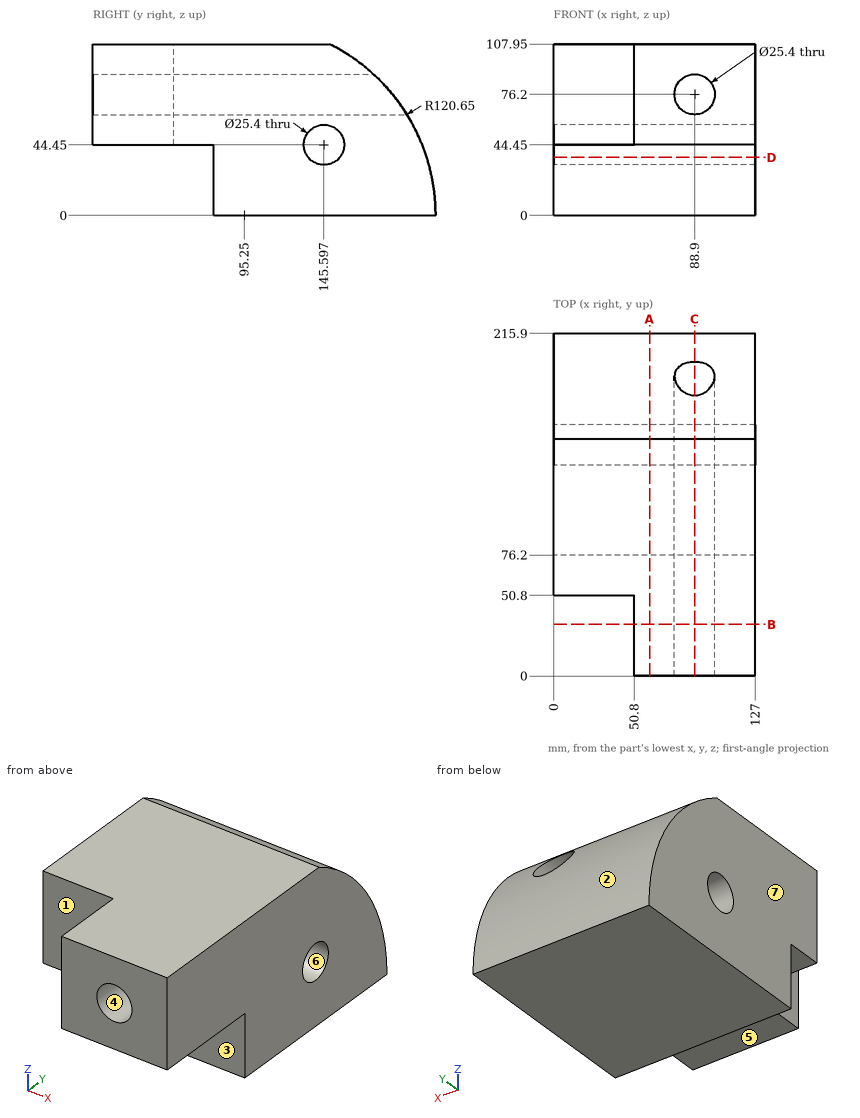
Job drawing, mm, ordinate dimensions from the low corner. One solid piece. A direction names the side the tool comes from. Round coordinates to 2 decimals unless told otherwise and drop trailing zeros. Order: outer loops, then holes, each group sorted by start corner. A loop starts at its lowest first (then second) coordinate and runs counter-clockwise, first axis right, second up. Notation, with made-up numbers: (-22, 54.25) -> (12, 54.25) arc R21 cw to (12, 61.25) -> close; hole circle Ø7 at (-5.5, -36). An arc over 180 degrees is marked (long way). Answer in a Markdown table with one row per item.
1) Mould opens along Z. For the marked faces 4, 5, 6 and 7 say: released by +Z, released by -Z, zero draft, split by the parting line, or undercut.
Values:
| item | result |
|---|---|
| face 4 | undercut |
| face 5 | released by -Z |
| face 6 | undercut |
| face 7 | zero draft |
2) Band-saw the part on A-A on x = 60.5. Give the cut face in (y, z).
Values:
| item | result |
|---|---|
| outline | (0, 44.45) -> (76.2, 44.45) -> (76.2, 0) -> (215.9, 0) arc R120.65 ccw to (149.13, 107.95) -> (0, 107.95) -> close; hole circle Ø25.4 at (145.6, 44.45) |
3) Band-saw the part on C-C on x = 88.9. Give the cut face in (y, z).
Values:
| item | result |
|---|---|
| outline | (0, 44.45) -> (76.2, 44.45) -> (76.2, 0) -> (215.9, 0) arc R120.65 ccw to (197.84, 63.5) -> (0, 63.5) -> close; (0, 88.9) -> (176.82, 88.9) arc R120.65 ccw to (149.13, 107.95) -> (0, 107.95) -> close; hole circle Ø25.4 at (145.6, 44.45) |
4) Band-saw the part on D-D on z = 36.5. Give the cut face in (x, y), and give its area (3 significant figures).
Values:
| item | result |
|---|---|
| outline | (0, 76.2) -> (127, 76.2) -> (127, 135.69) -> (0, 135.69) -> close; (0, 155.5) -> (127, 155.5) -> (127, 210.25) -> (0, 210.25) -> close |
| area | 14,500 mm2 |
5) Which spindle directions (+Z, -Z, +X, -X, +Y, -Y) get a long thin tool onto all of the face, cutting with end or side? Do the marked faces 1, 2 and 3. Say none if no direction does.
Values:
| item | result |
|---|---|
| face 1 | +Z, -Z, -X, -Y |
| face 2 | +Z, +X, -X, +Y |
| face 3 | -Z, +X, -X, -Y |
6) Wall check: L1, parallel to Z at x = 88.9, y = 114.5; L2, parallel to X at y = 25, z = 54.5; L3, parallel to X at y = 14, z = 69. Give the ranges that are in metal, low to high.
Values:
| item | result |
|---|---|
| L1 | 0 to 63.5, 88.9 to 107.95 |
| L2 | 50.8 to 127 |
| L3 | 50.8 to 78.44, 99.36 to 127 |
7) Pin check, flat tips, straight feed: P1, Ø15, axis at x = 34, z = 71, coming from the -Y side; P2, Ø23, axis at x = 78, y = 49.5, coming from the -Z side; P3, Ø4, axis at x = 75, z = 68, coming from the +Y side. Stop position of each tip, or through.
Values:
| item | result |
|---|---|
| P1 | y = 50.8 |
| P2 | z = 44.45 |
| P3 | y = 196.25 |
8) Band-saw the part on B-B on y = 32.5. Give the cut face in (x, z).
Values:
| item | result |
|---|---|
| outline | (50.8, 44.45) -> (127, 44.45) -> (127, 107.95) -> (50.8, 107.95) -> close; hole circle Ø25.4 at (88.9, 76.2) |
